```python
from build123d import *

# Parameters (mm, degrees)
F0_R      = 17.25
F0_R_2    = 14.25
F1_DEPTH  = 22
F0_R_3    = 5.25
F2_DEPTH  = 2
F0_R_4    = 1.85
F3_DEPTH  = 12
F5_DEPTH  = 34
F7_DEPTH  = 7.1787528205
F8_R      = 2.25
F10_DEPTH = 7.1787528205
F9_R      = 2.25
F11_DEPTH = 7.1787528205
F13_DEPTH = 25


with BuildPart() as f1:
    # F0 (on Right) → F1 (new body)
    with BuildSketch(Plane.YZ):
        Circle(F0_R)
        Circle(F0_R_2, mode=Mode.SUBTRACT)
    extrude(amount=F1_DEPTH)

    # F0 (on Right) → F2 (join)
    with BuildSketch(Plane.YZ):
        Circle(F0_R)
        Circle(F0_R_2, mode=Mode.SUBTRACT)
        Circle(F0_R_2)
        Circle(F0_R_3, mode=Mode.SUBTRACT)
    extrude(amount=F2_DEPTH)

    # F0 (on Right) → F3 (join)
    with BuildSketch(Plane.YZ):
        Circle(F0_R)
        Circle(F0_R_2, mode=Mode.SUBTRACT)
        Circle(F0_R_2)
        Circle(F0_R_3, mode=Mode.SUBTRACT)
        Circle(F0_R_3)
        Circle(F0_R_4, mode=Mode.SUBTRACT)
    extrude(amount=-F3_DEPTH)

    # F4 (on face) → F5 (join, through all)
    with BuildSketch(Plane(origin=(-12, 0, 0), x_dir=(0, -1, 0), z_dir=(-1, 0, 0))):
        with BuildLine():
            Line((-5, 20.25), (-5, 16.5094669811))
            ThreePointArc((-5, 16.5094669811), (2.2123277405, 17.1075452935), (9.0352533152, 14.6944444444))
            Line((9.0352533152, 14.6944444444), (0, 20.25))
            Line((0, 20.25), (-5, 20.25))
        make_face()
        with BuildLine():
            Line((-15.0370144266, -14.4551270189), (-11.7976178086, -12.5848605095))
            ThreePointArc((-11.7976178086, -12.5848605095), (-15.9217326908, -6.6378406219), (-17.243388841, 0.4775366783))
            Line((-17.243388841, 0.4775366783), (-17.5370144266, -10.125))
            Line((-17.5370144266, -10.125), (-15.0370144266, -14.4551270189))
        make_face()
        with BuildLine():
            Line((20.0370144266, -5.7948729811), (16.7976178086, -3.9246064716))
            ThreePointArc((16.7976178086, -3.9246064716), (13.7094049503, -10.4697046715), (8.2081355258, -15.1719811228))
            Line((8.2081355258, -15.1719811228), (17.5370144266, -10.125))
            Line((17.5370144266, -10.125), (20.0370144266, -5.7948729811))
        make_face()
    extrude(amount=-F5_DEPTH)

    # F6 (on face) → F7 (cut, up to face)
    with BuildSketch(Plane.XY.offset(20.25)):
        with BuildLine():
            ThreePointArc((4.75, 0), (7, -2.25), (9.25, 0))
            Line((9.25, 0), (4.75, 0))
        make_face()
        with BuildLine():
            Line((4.75, 0), (9.25, 0))
            ThreePointArc((9.25, 0), (7, 2.25), (4.75, 0))
        make_face()
    extrude(amount=-F7_DEPTH, mode=Mode.SUBTRACT)

    # F8 (on face) → F10 (cut, up to face)
    with BuildSketch(Plane(origin=(0, 17.5370144266, -10.125), x_dir=(-1, 0, 0), z_dir=(0, 0.8660254038, -0.5))):
        with Locations((-7, 0)):
            Circle(F8_R)
    extrude(amount=-F10_DEPTH, mode=Mode.SUBTRACT)

    # F9 (on face) → F11 (cut, up to face)
    with BuildSketch(Plane(origin=(0, -17.5370144266, -10.125), x_dir=(1, 0, 0), z_dir=(0, -0.8660254038, -0.5))):
        with Locations((7, 0)):
            Circle(F9_R)
    extrude(amount=-F11_DEPTH, mode=Mode.SUBTRACT)

    # F12 (on face) → F13 (cut)
    with BuildSketch(Plane(origin=(-12, 0, 0), x_dir=(0, -1, 0), z_dir=(-1, 0, 0))):
        with BuildLine():
            ThreePointArc((-4.8264703056, -0.4771628534), (-4.2002232084, 2.425), (-2, 4.418427322))
            Line((-2, 4.418427322), (-2, 12.0856319653))
            ThreePointArc((-2, 12.0856319653), (-10.6088111964, 6.125), (-11.4664643027, -4.3107651751))
            Line((-11.4664643027, -4.3107651751), (-4.8264703056, -0.4771628534))
        make_face()
        with BuildLine():
            ThreePointArc((2, 4.418427322), (4.0756901256, 2.6289256361), (4.85, 0))
            ThreePointArc((4.85, 0), (4.8441140048, -0.2388713227), (4.8264703056, -0.4771628534))
            Line((4.8264703056, -0.4771628534), (11.4664643027, -4.3107651751))
            ThreePointArc((11.4664643027, -4.3107651751), (12.0525243768, -2.1906976391), (12.25, 0))
            ThreePointArc((12.25, 0), (9.3424434705, 7.9234619959), (2, 12.0856319653))
            Line((2, 12.0856319653), (2, 4.418427322))
        make_face()
        with BuildLine():
            Line((9.4664643027, -7.7748667902), (2.8264703056, -3.9412644686))
            ThreePointArc((2.8264703056, -3.9412644686), (0, -4.85), (-2.8264703056, -3.9412644686))
            Line((-2.8264703056, -3.9412644686), (-9.4664643027, -7.7748667902))
            ThreePointArc((-9.4664643027, -7.7748667902), (0, -12.25), (9.4664643027, -7.7748667902))
        make_face()
    extrude(amount=-F13_DEPTH, mode=Mode.SUBTRACT)


solid = f1.part
```
Can you work these out from the model? Positions are in its coordinate system, mm. A direction names the side the tool comes from. Round coordinates to 2 decimals unless told otherwise and drop trailing zeros. Loops run counter-clockwise (first coordinate to the right, second up) from the corner with the lowest first, then second, coordinate; pieces in that order, holes last. Notation, with made-up numbers: M 27,19 L 46,19 A14 cw 46,36 Z; hole C -3,64.5 d3. An arc over 180 degrees is marked long. Write item = value, one per line. Start each with the question number.
(1) Suppose I cut it at D-D on y = 8.5. Write out the boundary of the cut face in (x, z).
(2) I need wall thicknesses on line 1 along Y through (x, z) = (13, 0); line 2 along Y through (x, z) = (-9, 7.5); line 3 along Z through (x, y) = (4.5, -12.5). Which ranges of each line are inside material? Lowest first, please.
(3) Suppose I cut it at B-B on z = 10.5. Write out the boundary of the cut face in (x, y).
(4) Suppose I cut it at C-C on x = 11.5. Write out the boundary of the cut face in (y, z) (3 decimals), plus the area to 3 significant figures.
(5) I'm going to push flat-ended pins straight in: P1, Ø8.5, axis at x = -6, z = 8.5, coming from the +Y side; P2, Ø4, axis at x = 12, z = 18, coming from the +Y side; P3, Ø5, axis at x = 4, y = -8, coming from the -Z side; P4, Ø2, axis at y = 0, z = 0, coming from the +X side. Where does each tip first touch, or does it pass through?
(6) Which directions (+Z, -Z, +X, -X, +Y, -Y) give clear straight access to the entire face, cutting with the end or side of a thin tool? Please do faces 5 (the face through (0, -0.1, -2)), 6 (the face through (4.762, 13.44, -13.533)), 7 (the face through (5, 2, 20.25)), 8 (the face through (-5.098, -6.193, -5.885)), 9 (the face through (4.762, -4.581, 17.433)).
(7) If we mould it in two halves opening along Y, with no side actions, what happens to faces 1 (the face through (-5.1, 10.53, 6.26)), 2 (the face through (5.24, 13.8, 10.35)), 3 (the face through (22, 4, -14)), 4 (the face through (-6.08, 4.22, 2.39))? For each: released by +Y, released by -Y, zero draft, split by the parting line, or undercut.
(8) Suppose I cut it at A-A on x = -8. Write out the boundary of the cut face in (y, z) (3 decimals).
Answer block:
q1.outline = M -12,-15.01 L 22,-15.01 L 22,-11.44 L 2,-11.44 L 2,-8.82 L -12,-8.82 Z; M -12,-7.22 L 2,-7.22 L 2,-2.6 L -12,-2.6 Z; M -12,8.82 L 2,8.82 L 2,11.44 L 22,11.44 L 22,15.01 L -12,15.01 Z
q2.line_1 = -17.25 to -14.25, 14.25 to 17.26
q2.line_2 = -15.53 to -9.69, -2 to 2, 9.69 to 15.53
q2.line_3 = -12.85 to -6.84, 6.84 to 11.89
q3.outline = M -12,-13.69 L 22,-13.69 L 22,-9.63 L 2,-9.63 L 2,-6.31 L -12,-6.31 Z; M -12,-2 L 2,-2 L 2,2 L -12,2 Z; M -12,6.31 L 2,6.31 L 2,9.63 L 22,9.63 L 22,13.69 L -12,13.69 Z
q4.outline = M -20.037,-5.795 L -17.537,-10.125 L -8.208,-15.172 A17.25 ccw 11.798,-12.585 L 15.037,-14.455 L 17.537,-10.125 L 17.243,0.478 A17.25 ccw 5,16.509 L 5,20.25 L 0,20.25 L -9.035,14.694 A17.25 ccw -16.798,-3.925 Z; hole C 0,0 d28.5
q4.area = 374 mm²
q5.P1 = 16.72
q5.P2 = 6.45
q5.P3 = -16.35
q5.P4 = through
q6.face_5 = +X
q6.face_6 = -Z, +X, -X
q6.face_7 = +Z, +X, -X, +Y, -Y
q6.face_8 = +X, -X
q6.face_9 = +Z, +X, -X, -Y
q7.face_1 = undercut
q7.face_2 = released by +Y
q7.face_3 = zero draft
q7.face_4 = undercut
q8.outline = M -20.037,-5.795 L -17.537,-10.125 L -8.208,-15.172 A17.25 ccw 11.798,-12.585 L 15.037,-14.455 L 17.537,-10.125 L 17.243,0.478 A17.25 ccw 5,16.509 L 5,20.25 L 0,20.25 L -9.035,14.694 A17.25 ccw -16.798,-3.925 Z; hole M -11.466,-4.311 L -4.826,-0.477 A4.85 cw -2,4.418 L -2,12.086 A12.25 ccw Z; hole M -9.466,-7.775 A12.25 ccw 9.466,-7.775 L 2.826,-3.941 A4.85 cw -2.826,-3.941 Z; hole C 0,0 d3.7; hole M 2,4.418 A4.85 cw 4.826,-0.477 L 11.466,-4.311 A12.25 ccw 2,12.086 Z
